from build123d import *

# Parameters (mm, degrees)
F4_DEPTH = 25


with BuildPart() as f2:
    # F0 (on Front) → F2 (revolve)
    with BuildSketch(Plane.XZ):
        with BuildLine():
            Line((-13.726478, 5), (-19.509004, 5))
            ThreePointArc((-19.509004, 5), (-19.784693, 4.961247), (-20.039014, 4.847991))
            Line((-20.039014, 4.847991), (-23.117382, 2.923956))
            ThreePointArc((-23.117382, 2.923956), (-23.352377, 2.499956), (-23.117375, 2.07596))
            Line((-23.117375, 2.07596), (-20.039018, 0.152))
            ThreePointArc((-20.039018, 0.152), (-19.784703, 0.038751), (-19.509022, 0))
            Line((-19.509022, 0), (-13.726467, 0))
            ThreePointArc((-13.726467, 0), (-13.345413, 0.075447), (-13.021858, 0.290404))
            Line((-13.021858, 0.290404), (-11.511276, 1.79037))
            ThreePointArc((-11.511276, 1.79037), (-11.215885, 2.499957), (-11.511263, 3.209549))
            Line((-11.511263, 3.209549), (-13.021856, 4.709582))
            ThreePointArc((-13.021856, 4.709582), (-13.345416, 4.924549), (-13.726478, 5))
        make_face()
    revolve(axis=Axis((0, 0, 36.743954), (0, 0, 1)))

    # F3 (on Top) → F4 (cut)
    with BuildSketch(Plane.XY):
        Polygon((2.5, 18.654833), (-2.5, 18.654833), (0, 14.324706), align=None)
        Polygon((-12.40556, -7.162353), (-17.40556, -7.162353), (-14.90556, -11.49248), align=None)
        Polygon((12.40556, -7.162353), (14.90556, -11.49248), (17.40556, -7.162353), align=None)
    extrude(amount=F4_DEPTH, mode=Mode.SUBTRACT)


solid = f2.part
Verification items for the finished model (mm, model axes). A direction names the side the tool comes from. Give positions to 0.01 mm unless a question says otherwise; leave off trailing zeros. Write each loop counter-clockwise with the first axis right and the second up, starting at its lowest first coordinate (ties: lowest second). Pieces come first, ordered by that corner, then holes.
(1) Gauge pin test, flat ends, axial feed: pin 1 (2.5 mm diameter, centred on x = -1, z = 2, fed in from -Y); pin 2 (1 mm diameter, centred on x = -3.5, z = 3.5, fed in from -Y); pin 3 (1.5 mm diameter, centred on y = -11.5, z = 4, fed in from -X). Record the tip position at first contact, or that the pin passes through.
(2) Cross-section at A-A (y = 0). Enter the section's corners in (x, z).
(3) Material ranges on line 1 (Y direction, x = 1, z = 3.9); line 2 (Y direction, x = -9, z = 3.7); line 3 (X direction, y = 4, z = 4.3), recorded low to high.
(4) Access from +Z, -Z, +X, -X, +Y, -Y to the whole of each face (thin tool, end or side, straight path). Record for faces 4 (the face through (16.138, -9.358, 2.465)), 5 (the face through (16.021, 12.284, 0.245)).
(5) Mould release check, pull along Y, two halves, no side actions. Record for faces 1 (the face through (4.386, 19.75, 4.728)), 2 (the face through (-4.1, -13.3, 0)), 3 (the face through (1.233, 16.459, 2.465)): +Y half, -Y half, draft (parallel to the pull), parting line (faces both ways), or undercut.
Worked out:
1. pin 1: stops at y = -23.35
1. pin 2: stops at y = -22.73
1. pin 3: stops at x = -19.52
2. outline: (-23.12, 2.08) - (-20.04, 0.15) arc R1 ccw to (-19.51, 0) - (-13.73, 0) arc R1 ccw to (-13.02, 0.29) - (-11.51, 1.79) arc R1 ccw to (-11.51, 3.21) - (-13.02, 4.71) arc R1 ccw to (-13.73, 5) - (-19.51, 5) arc R1 ccw to (-20.04, 4.85) - (-23.12, 2.92) arc R0.5 ccw to start; (11.51, 1.79) - (13.02, 0.29) arc R1 ccw to (13.73, 0) - (19.51, 0) arc R1 ccw to (20.04, 0.15) - (23.12, 2.08) arc R0.5 ccw to (23.12, 2.92) - (20.04, 4.85) arc R1 ccw to (19.51, 5) - (13.73, 5) arc R1 ccw to (13.02, 4.71) - (11.51, 3.21) arc R1 ccw to start
3. line 1: y = -21.53 to -12.17, 12.17 to 16.06, 18.65 to 21.53
3. line 2: y = -19.94 to -7.95, 7.95 to 19.94
3. line 3: x = -20.53 to -11.96, 11.96 to 20.53
4. face 4: +Z, -Z
4. face 5: -Z
5. face 1: parting line
5. face 2: draft
5. face 3: undercut
